from build123d import *

# Parameters (mm, degrees)
EXTRUDE_THIN1_DEPTH = 134.9375
FILLET1_R           = 1.016


with BuildPart() as part:
    # Sketch1 → Extrude-Thin1 (new body)
    with BuildSketch(Plane.XY):
        with BuildLine():
            Line((0, 0), (-9.525, 0))
            Line((-9.525, 0), (-9.525, 6.35))
            Line((-9.525, 6.35), (-7.14375, 6.35))
            ThreePointArc((-7.14375, 6.35), (-5.051394068, 11.401394068), (0, 13.49375))
            Line((0, 13.49375), (0, 12.47775))
            ThreePointArc((0, 12.47775), (-4.678413944, 10.30749454), (-6.042935054, 5.334))
            Line((-6.042935054, 5.334), (-8.509, 5.334))
            Line((-8.509, 5.334), (-8.509, 1.016))
            Line((-8.509, 1.016), (0, 1.016))
            Line((0, 1.016), (0, 0))
        make_face()
    extrude(amount=-EXTRUDE_THIN1_DEPTH)

    # Fillet1
    fillet1_edges = [part.edges().sort_by_distance(p)[0] for p in [
        (-6.042935054, 5.334, -67.46875),
        (-9.525, 0, -67.46875),
        (-9.525, 6.35, -67.46875),
    ]]
    fillet(fillet1_edges, radius=FILLET1_R)


solid = part.part
Can you work these out from the model? Positions are in its coordinate system, mm. A direction names the side the tool comes from. Round coordinates to 2 decimals unless told otherwise and drop trailing zeros. Loops run counter-clockwise (first coordinate to the right, second up) from the corner with the lowest first, then second, coordinate; pieces in that order, holes last. Notation, with made-up numbers: (-11, -31.75) - (41, -31.75) arc R21 cw to (41, -23.75) - close; hole circle Ø7 at (-30, 21.25). An arc over 180 degrees is marked (long way). Answer in a Markdown table with one row per item. Add a question column.
Q1. I want a section at C-C on y = 2.25. List the corners of the cut face in (x, z) for me (1 decimal).
Q2. Which directions (+Z, -Z, +X, -X, +Y, -Y) give clear straight access to the entire face, cutting with the end or side of a thin tool? Please do faces 4 (the flat face through (-8.509, 3, -67)), 5 (the flat face through (-7, 6, -134.938)).
Q3. I want a section at A-A on x = -3.75. List the corners of the cut face in (y, z) for me.
Q4. I need wall thicknesses on L1, parallel to Y at x = -7.25, z = -6.5; L2, parallel to Y at x = -0.25, z = -51.5; L3, parallel to X at y = 5, z = -94 (3 decimals). Which ranges of each line are inside material? Lowest first, please.
Q5. For pin 1 Ø1.1 at (x, z) = (-8, -54) entering from +Y; pin 2 Ø2.5 at (x, z) = (-4.5, -65) entering from +Y; pin 3 Ø2 at (x, z) = (-5.5, -106) entering from +Y; pin 4 Ø1.5 at (y, z) = (5.5, -63.5) entering from -X (3 decimals), each with a flat end and sliding along its axis, tell me the tip position at first contact or that it passes through.
Q6. We'd pull the mould along Y, two halves only. Please class faces 1 (the cylindrical face through (-4.285, 10.73, -66.524)), 2 (the flat face through (-9.525, 3, -67)), 3 (the cylindrical face through (-5.107, 11.346, -66.524)): pulls with the +Y half, pulls with the -Y half, needs draft (parallel to the pull), parting line crosses it, or undercut.
A:
| question | item | result |
|---|---|---|
| 1 | outline | (-9.5, -134.9) - (-8.5, -134.9) - (-8.5, 0) - (-9.5, 0) - close |
| 2 | face 4 | +Z, -Z, +X |
| 2 | face 5 | -Z, +X, -X, +Y, -Y |
| 3 | outline | (0, -134.94) - (1.02, -134.94) - (1.02, 0) - (0, 0) - close; (11.2, -134.94) - (12.43, -134.94) - (12.43, 0) - (11.2, 0) - close |
| 4 | L1 | 0 to 1.02, 5.33 to 6.35 |
| 4 | L2 | 0 to 1.02, 12.47 to 13.49 |
| 4 | L3 | -9.525 to -8.509 |
| 5 | pin 1 | y = 6.35 |
| 5 | pin 2 | y = 12.71 |
| 5 | pin 3 | y = 11.9 |
| 5 | pin 4 | x = -9.525 |
| 6 | face 1 | undercut |
| 6 | face 2 | needs draft |
| 6 | face 3 | pulls with the +Y half |
